Read the model definition and answer for the solid it produces. Units are mm, in the model's axes. A direction names the side the tool comes from. Coordinates: 2 decimals unless noted, no trailing zeros. Write each loop counter-clockwise with the first axis right and the second up, starting at its lowest first coordinate (ties: lowest second). Pieces come first, ordered by that corner, then holes.
(1) Find the intervals of material crossed by probe 1 along Y at (x, z) = (3.5, 2.75); probe 2 along Z at (x, y) = (1.25, 12); probe 3 along X at (y, z) = (2, 5), in increasing order.
(2) Given pin 1 (1.5 mm diameter, centred on y = 62.5, z = 6.5, fed in from +X); pin 2 (1.8 mm diameter, centred on y = 78, z = 7, fed in from +X); pin 3 (2 mm diameter, centred on y = 70.5, z = 11, fed in from -X); pin 4 (0.5 mm diameter, centred on x = 3.5, y = 4.5, fed in from +Z), each flat-ended and moving along its own axis, determine where each tip first touches the part or whether it passes through.
(3) Section A-A on z = -0.75 is taken. Write down the section's boundary in (x, y), then the cut area to 3 significant figures.
(4) Section B-B on y = 9 is taken. Write down the section's boundary in (x, z).
(5) Section C-C on z = 3.25 is taken. Write down the section's boundary in (x, y), then the cut area to 3 significant figures.
(6) The mould has two halves that part along Y. Classify faces 4 (the cylindrical face through (12, 60, 7)), 5 (the flat face through (0, 27, 6)), 6 (the flat face through (22, 75, 7)), 7 (the flat face through (22, 63, 7)): +Y half, -Y half, draft (parallel to the pull), parting line (faces both ways), or undercut.
(7) Which of the six approach directions +Z, -Z, +X, -X, +Y, -Y give full straight-line access (tool end or side, diameter ignored) to faces 1 (the flat face through (24, 67, 7)), 2 (the flat face through (10, 20, 6)), 3 (the flat face through (5, 13, -1))?
(8) Section D-D on x = 15.75 is taken. Write down the section's boundary in (y, z), then the cut area to 3 significant figures.
Autodesk Fusion 360 part; units mm, degrees
sketch "Sketch1" plane through (0, 0, 0) normal (1, 0, 0) x (0, 1, 0)
  line L0 (0, 0) -> (0, 5) construction
  line L1 (0, 5) -> (3, 5) construction
  line L2 (3, 5) -> (3, 0) construction
  line L3 (3, 0) -> (0, 0) construction
  line L4 (0, 5) -> (-2, 5) construction
  line L5 (-2, 5) -> (-2, 9) construction
  line L6 (0, 0) -> (-2, 0) construction
  line L7 (-2, 0) -> (-2, -3) construction
  line L8 (-2, -3) -> (5, -3) construction
  line L9 (5, -3) -> (5, 0) construction
  line L10 (5, 0) -> (3, 0) construction
  line L11 (3, 5) -> (5, 5) construction
  line L12 (5, 5) -> (5, 9) construction
  line L13 (-2, 9) -> (5, 9) construction
  line L14 (-2, 5) -> (0, 5)
  line L15 (0, 5) -> (0, 0)
  line L16 (0, 0) -> (-2, 0)
  line L17 (-2, 0) -> (-2, -3)
  line L18 (-2, -3) -> (5, -3)
  line L19 (5, -3) -> (5, 0)
  line L20 (5, 0) -> (3, 0)
  line L21 (3, 0) -> (3, 5)
  line L22 (3, 5) -> (5, 5)
  line L23 (5, 5) -> (5, 9)
  line L24 (5, 9) -> (-2, 9)
  line L25 (-2, 9) -> (-2, 5)
  line L26 (-2, 5) -> (0, 5)
  line L27 (5, 9) -> (-2, 9)
  line L28 (-2, 0) -> (-2, -3)
  line L29 (3, 5) -> (5, 5) construction
  line L30 (5, 5) -> (5, 9) construction
  line L31 (5, 0) -> (3, 0)
  line L32 (-2, 0) -> (-2, -3) construction
  line L33 (5, 0) -> (3, 0) construction
  line L34 (-2, 9) -> (5, 9) construction
  line L35 (-2, -3) -> (5, -3) construction
  line L36 (-2, -3) -> (5, -3)
  line L37 (-2, 9) -> (-2, 5)
  line L38 (5, -3) -> (5, 0) construction
  line L39 (3, 5) -> (3, 0) construction
  line L40 (5, -3) -> (5, 0)
  line L41 (0, 0) -> (-2, 0)
  line L42 (3, 0) -> (3, 5)
  line L43 (0, 0) -> (-2, 0) construction
  line L44 (-2, 5) -> (-2, 9) construction
  line L45 (0, 5) -> (3, 5) construction
  line L46 (3, 5) -> (5, 5)
  line L47 (5, 5) -> (5, 9)
  line L48 (0, 0) -> (0, 5) construction
  line L49 (3, 0) -> (0, 0) construction
  line L50 (0, 5) -> (-2, 5) construction
  line L51 (0, 5) -> (0, 0)
  line L52 (13, 5) -> (15, 5)
  line L53 (20, 9) -> (13, 9)
  line L54 (13, 0) -> (13, -3)
  line L55 (18, 5) -> (20, 5) construction
  line L56 (20, 5) -> (20, 9) construction
  line L57 (20, 0) -> (18, 0)
  line L58 (13, 0) -> (13, -3) construction
  line L59 (20, 0) -> (18, 0) construction
  line L60 (13, 9) -> (20, 9) construction
  line L61 (13, -3) -> (20, -3) construction
  line L62 (13, -3) -> (20, -3)
  line L63 (13, 9) -> (13, 5)
  line L64 (20, -3) -> (20, 0) construction
  line L65 (18, 5) -> (18, 0) construction
  line L66 (20, -3) -> (20, 0)
  line L67 (15, 0) -> (13, 0)
  line L68 (18, 0) -> (18, 5)
  line L69 (15, 0) -> (13, 0) construction
  line L70 (13, 5) -> (13, 9) construction
  line L71 (15, 5) -> (18, 5) construction
  line L72 (18, 5) -> (20, 5)
  line L73 (20, 5) -> (20, 9)
  line L74 (15, 0) -> (15, 5) construction
  line L75 (18, 0) -> (15, 0) construction
  line L76 (15, 5) -> (13, 5) construction
  line L77 (15, 5) -> (15, 0)
  point P0 (15, 0)
  dimension "d1" = 5
  dimension "d2" = 3
  dimension "d3" = 2
  dimension "d4" = 4
  dimension "d5" = 3
  dimension "d6" = 2
  dimension "d7" = 4
  dimension "d8" = 5
  dimension "d9" = 3
  dimension "d10" = 2
  dimension "d11" = 4
  dimension "d12" = 3
  dimension "d13" = 2
  dimension "d14" = 4
  dimension "d15" = 5
  dimension "d16" = 3
  dimension "d17" = 2
  dimension "d18" = 4
  dimension "d19" = 3
  dimension "d20" = 2
  dimension "d21" = 4
extrude "Extrude1" add sketch "Sketch1" along normal blind 10 makes body 1 at (6.6667, 0.3333, -3) makes body 2 at (3.3333, 15.3333, -3)
extrude "Extrude2" add 1 faces at (3.3333, 5, 6.3333) along direction (0, 1, 0) blind 8 on bodies 1 bodies 1 2
fillet "Fillet1" radius 1 1 edges at (5, 18, 5) on bodies 1
fillet "Fillet2" radius 1 1 edges at (5, 18, 0) on bodies 1
fillet "Fillet3" radius 1 1 edges at (5, 15, 0) on bodies 1
fillet "Fillet4" radius 1 1 edges at (5, 15, 5) on bodies 1
fillet "Fillet5" radius 1 1 edges at (5, 3, 0) on bodies 1
fillet "Fillet6" radius 1 1 edges at (5, 0, 0) on bodies 1
fillet "Fillet7" radius 1 1 edges at (5, 0, 5) on bodies 1
fillet "Fillet8" radius 1 1 edges at (5, 3, 5) on bodies 1
extrude "Extrude3" add 1 faces at (3.3333, 20, 6.3333) along direction (0, 1, 0) blind 59 on bodies 1 bodies 1
sketch "Sketch2" plane through (0, 0, 9) normal (0, 0, 1) x (-1, 0, 0)
  line L0 (0, -5) -> (-10, -5)
  line L1 (-10, -5) -> (-10, -13)
  line L2 (-10, -13) -> (0, -13)
  line L3 (0, -13) -> (0, -5)
  line L4 (-5, -13) -> (-5, -9) construction
  circle A0 centre (-5, -9) radius 2.5
  dimension "d44" = 5
extrude "Extrude4" add sketch "Sketch2" along normal blind 5 contours A0 bodies 1
sketch "Sketch3" plane through (10, 0, 0) normal (1, 0, 0) x (0, 1, 0)
  line L0 (0, 4) -> (0, 1)
  arc A0 (-1, 0) -> (0, 1) centre (-1, 1) ccw
  line L1 (-1, 0) -> (-2, 0)
  line L2 (-2, 0) -> (-2, -3)
  line L3 (-2, -3) -> (5, -3)
  line L4 (5, -3) -> (5, 0)
  line L5 (5, 0) -> (4, 0)
  arc A1 (3, 1) -> (4, 0) centre (4, 1) ccw
  line L6 (3, 1) -> (3, 4)
  arc A2 (4, 5) -> (3, 4) centre (4, 4) ccw
  line L7 (4, 5) -> (14, 5)
  arc A3 (15, 4) -> (14, 5) centre (14, 4) ccw
  line L8 (15, 4) -> (15, 1)
  arc A4 (14, 0) -> (15, 1) centre (14, 1) ccw
  line L9 (14, 0) -> (13, 0)
  line L10 (13, 0) -> (13, -3)
  line L11 (13, -3) -> (20, -3)
  line L12 (20, -3) -> (20, 0)
  line L13 (20, 0) -> (19, 0)
  arc A5 (18, 1) -> (19, 0) centre (19, 1) ccw
  line L14 (18, 1) -> (18, 4)
  arc A6 (19, 5) -> (18, 4) centre (19, 4) ccw
  line L15 (19, 5) -> (79, 5)
  line L16 (79, 5) -> (79, 9)
  line L17 (79, 9) -> (20, 9)
  line L18 (20, 9) -> (13, 9)
  line L19 (13, 9) -> (5, 9)
  line L20 (5, 9) -> (-2, 9)
  line L21 (-2, 9) -> (-2, 5)
  line L22 (-2, 5) -> (-1, 5)
  arc A7 (0, 4) -> (-1, 5) centre (-1, 4) ccw
  line L23 (79, 5) -> (61, 5)
  line L24 (61, 5) -> (61, 9)
  line L25 (61, 9) -> (79, 9)
  line L26 (79, 9) -> (79, 5)
  dimension "d47" = 18
extrude "Extrude5" add sketch "Sketch3" along normal blind 14 contours L15 L16 L17 L23 L24 L25 L26 bodies 1
fillet "Fillet9" radius 5 1 edges at (10, 61, 7) on bodies 1
fillet "Fillet10" radius 5 1 edges at (0, 79, 7) on bodies 1
sketch "Sketch4" plane through (0, 0, 9) normal (0, 0, 1) x (-1, 0, 0)
  arc A0 (-5, -79) -> (0, -74) centre (-5, -74) ccw
  line L0 (0, -74) -> (0, -20)
  line L1 (0, -20) -> (-10, -20)
  line L2 (-10, -20) -> (-10, -56)
  arc A1 (-15, -61) -> (-10, -56) centre (-15, -56) ccw
  line L3 (-15, -61) -> (-24, -61)
  line L4 (-24, -61) -> (-24, -79)
  line L5 (-24, -79) -> (-5, -79)
  line L6 (-22, -79) -> (-26, -79) construction
  line L7 (-26, -79) -> (-26, -61) construction
  line L8 (-26, -61) -> (-22, -61) construction
  line L9 (-22, -61) -> (-22, -79) construction
  line L10 (-26, -79) -> (-26, -77) construction
  line L11 (-26, -77) -> (-22, -76) construction
  line L12 (-22, -74) -> (-26, -73) construction
  line L13 (-26, -71) -> (-22, -70) construction
  line L14 (-22, -68) -> (-26, -67) construction
  line L15 (-26, -65) -> (-22, -64) construction
  line L16 (-22, -62) -> (-26, -61) construction
  line L17 (-26, -77) -> (-26, -77.5) construction
  line L18 (-22, -76) -> (-22, -76.5) construction
  line L19 (-26, -79) -> (-25.5, -79) construction
  line L20 (-26, -77.5) -> (-22, -76.5) construction
  line L21 (-25.5, -79) -> (-25.5, -77.375) construction
  line L22 (-26, -73) -> (-26, -72.5) construction
  line L23 (-22, -73.5) -> (-26, -72.5) construction
  line L24 (-26, -71.5) -> (-22, -70.5) construction
  line L25 (-22, -67.5) -> (-26, -66.5) construction
  line L26 (-22, -64.5) -> (-26, -65.5) construction
  line L27 (-22, -61.5) -> (-26, -60.5) construction
  line L28 (-25.5009, -60.6248) -> (-25.5009, -61.1248) construction
  line L29 (-25.5, -79) -> (-25.5, -77.375)
  line L30 (-25.5, -77.375) -> (-22, -76.5)
  line L31 (-25.5, -72.625) -> (-25.5, -71.375)
  line L32 (-22, -73.5) -> (-25.5, -72.625)
  line L33 (-25.5, -71.375) -> (-22, -70.5)
  line L34 (-25.5022, -66.6245) -> (-25.5022, -65.3756)
  line L35 (-22, -67.5) -> (-25.5022, -66.6245)
  line L36 (-22, -64.5) -> (-25.5022, -65.3756)
  line L37 (-22, -61.5) -> (-24.0719, -61)
  line L38 (-25.5, -79) -> (-22, -79)
  line L39 (-22, -79) -> (-22, -76.5)
  line L40 (-22, -73.5) -> (-22, -70.5)
  line L41 (-22, -67.5) -> (-22, -64.5)
  line L42 (-22, -61.5) -> (-22, -61)
  line L43 (-22, -61) -> (-24, -61)
  line L44 (-22, -70.5) -> (-22, -67.5)
  line L45 (-24, -71) -> (-24, -67)
  line L46 (-24, -65) -> (-24, -61)
  line L47 (-22, -64.5) -> (-22, -61.5)
  line L48 (-22, -76.5) -> (-22, -73.5)
  line L49 (-24, -77) -> (-24, -73)
  dimension "d54" = 0.5
  dimension "d55" = 0.5
extrude "Extrude6" add sketch "Sketch4" against normal blind 4 contours L4 L29 L30 L38 | L4 L31 L32 L33 | L4 L34 L35 L36 bodies 1
extrude "Extrude7" cut sketch "Sketch4" against normal blind 4 contours L4 L30 L32 L48 L49 | L4 L33 L35 L44 L45 | L4 L36 L37 L46 L47 bodies 1
Response:
1. probe 1: y = 0 to 3, 15 to 18
1. probe 2: z = 5 to 9
1. probe 3: x = 0 to 10
2. pin 1: stops at x = 22
2. pin 2: stops at x = 25.5
2. pin 3: passes through
2. pin 4: stops at z = 9
3. outline: (0, -2) - (10, -2) - (10, 5) - (0, 5) - close; (0, 13) - (10, 13) - (10, 20) - (0, 20) - close
3. area: 140 mm2
4. outline: (0, 5) - (10, 5) - (10, 9) - (7.5, 9) - (7.5, 14) - (2.5, 14) - (2.5, 9) - (0, 9) - close
5. outline: (0, 0) - (10, 0) - (10, 3) - (0, 3) - close; (0, 15) - (10, 15) - (10, 18) - (0, 18) - close
5. area: 60.0 mm2
6. face 4: -Y half
6. face 5: draft
6. face 6: undercut
6. face 7: undercut
7. face 1: +Z, -Z, +X
7. face 2: +Z, -Z, +X, -Y
7. face 3: -Z, +X, -X
8. outline: (61, 5) - (79, 5) - (79, 9) - (61, 9) - close
8. area: 72.0 mm2
